Geometry check sheet. Reference: the model listing, model coordinates, mm. Coordinates: 2 decimals unless noted, no trailing zeros. Loops run counter-clockwise (first coordinate to the right, second up) from the corner with the lowest first, then second, coordinate; pieces in that order, holes last. Notation, with made-up numbers: (81.25, 34) - (112.25, 34) arc R12 cw to (112.25, 57) - close; hole circle Ø5 at (2.5, -29.75). An arc over 180 degrees is marked (long way). One line per item, written item: value.
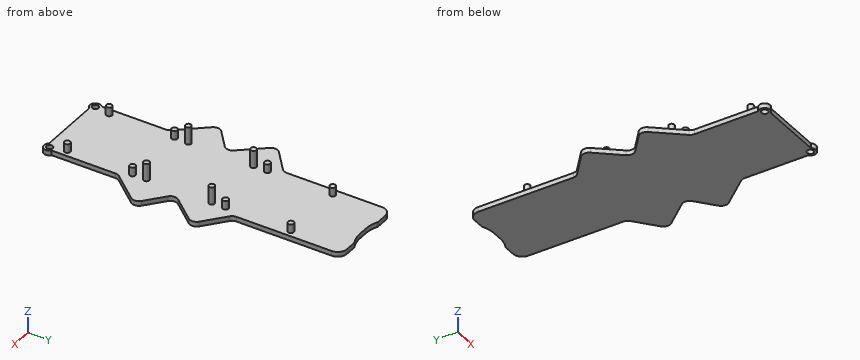
from build123d import *

# Parameters (mm, degrees)
F0_R     = 1.4859
F1_DEPTH = 2.2098
F2_R     = 1.33
F3_DEPTH = 4
F4_DEPTH = 8


with BuildPart() as f1:
    # F0 (on Top) → F1 (new body)
    with BuildSketch(Plane.XY):
        with BuildLine():
            Line((2.114807, 67.46875), (-2.114807, 67.46875))
            ThreePointArc((-2.114807, 67.46875), (-5.0139, 67.776541), (-7.783739, 68.686193))
            Line((-7.783739, 68.686193), (-8.215857, 68.880768))
            ThreePointArc((-8.215857, 68.880768), (-8.47063, 68.964439), (-8.737292, 68.99275))
            Line((-8.737292, 68.99275), (-13.69695, 68.99275))
            ThreePointArc((-13.69695, 68.99275), (-16.750237, 67.728037), (-18.01495, 64.67475))
            Line((-18.01495, 64.67475), (-18.01495, 20.943534))
            ThreePointArc((-18.01495, 20.943534), (-18.312512, 19.601529), (-19.149422, 18.511071))
            Line((-19.149422, 18.511071), (-28.620485, 10.56605))
            ThreePointArc((-28.620485, 10.56605), (-29.742839, 8.410727), (-29.01242, 6.09306))
            Line((-29.01242, 6.09306), (-20.055478, -4.584288))
            ThreePointArc((-20.055478, -4.584288), (-19.325058, -6.901955), (-20.447412, -9.057278))
            Line((-20.447412, -9.057278), (-28.620485, -15.91345))
            ThreePointArc((-28.620485, -15.91345), (-29.742839, -18.068773), (-29.01242, -20.38644))
            Line((-29.01242, -20.38644), (-18.757488, -32.611089))
            ThreePointArc((-18.757488, -32.611089), (-18.206354, -33.565901), (-18.01495, -34.651617))
            Line((-18.01495, -34.651617), (-18.01495, -63.949145))
            ThreePointArc((-18.01495, -63.949145), (-15.313338, -63.63877), (-13.864863, -65.940283))
            ThreePointArc((-13.864863, -65.940283), (-13.995237, -66.745649), (-14.373042, -67.46875))
            Line((-14.373042, -67.46875), (14.373042, -67.46875))
            ThreePointArc((14.373042, -67.46875), (14.643616, -64.104693), (18.01495, -63.949145))
            Line((18.01495, -63.949145), (18.01495, -34.651617))
            ThreePointArc((18.01495, -34.651617), (18.206354, -33.565901), (18.757488, -32.611089))
            Line((18.757488, -32.611089), (29.01242, -20.38644))
            ThreePointArc((29.01242, -20.38644), (29.742839, -18.068773), (28.620485, -15.91345))
            Line((28.620485, -15.91345), (20.447412, -9.057278))
            ThreePointArc((20.447412, -9.057278), (19.325058, -6.901955), (20.055478, -4.584288))
            Line((20.055478, -4.584288), (29.01242, 6.09306))
            ThreePointArc((29.01242, 6.09306), (29.742839, 8.410727), (28.620485, 10.56605))
            Line((28.620485, 10.56605), (19.149422, 18.511071))
            ThreePointArc((19.149422, 18.511071), (18.312512, 19.601529), (18.01495, 20.943534))
            Line((18.01495, 20.943534), (18.01495, 64.67475))
            ThreePointArc((18.01495, 64.67475), (16.750237, 67.728037), (13.69695, 68.99275))
            Line((13.69695, 68.99275), (8.737292, 68.99275))
            ThreePointArc((8.737292, 68.99275), (8.47063, 68.964439), (8.215857, 68.880768))
            Line((8.215857, 68.880768), (7.783739, 68.686193))
            ThreePointArc((7.783739, 68.686193), (5.0139, 67.776541), (2.114807, 67.46875))
        make_face()
        with BuildLine():
            ThreePointArc((-13.864863, -65.940283), (-15.313338, -63.63877), (-18.01495, -63.949145))
            ThreePointArc((-18.01495, -63.949145), (-18.19151, -67.775873), (-14.373042, -67.46875))
            ThreePointArc((-14.373042, -67.46875), (-13.995237, -66.745649), (-13.864863, -65.940283))
        make_face()
        with Locations((-16.417563, -65.940283)):
            Circle(F0_R, mode=Mode.SUBTRACT)
        with BuildLine():
            ThreePointArc((18.970263, -65.940283), (18.719076, -64.836058), (18.01495, -63.949145))
            ThreePointArc((18.01495, -63.949145), (14.643616, -64.104693), (14.373042, -67.46875))
            ThreePointArc((14.373042, -67.46875), (17.222929, -68.362609), (18.970263, -65.940283))
        make_face()
        with Locations((16.417563, -65.940283)):
            Circle(F0_R, mode=Mode.SUBTRACT)
    extrude(amount=F1_DEPTH)

    # F2 (on face) → F3 (join)
    with BuildSketch(Plane.XY.offset(2.2098)):
        with Locations((-15, 44.01575)):
            Circle(F2_R)
        with Locations((15, 44.01575)):
            Circle(F2_R)
        with Locations((15, 14.01575)):
            Circle(F2_R)
        with Locations((-15, 14.01575)):
            Circle(F2_R)
        with Locations((15, -28.68425)):
            Circle(F2_R)
        with Locations((-15, -28.68425)):
            Circle(F2_R)
        with Locations((-15, -58.68425)):
            Circle(F2_R)
        with Locations((15, -58.68425)):
            Circle(F2_R)
    extrude(amount=F3_DEPTH)

    # F2 (on face) → F4 (join)
    with BuildSketch(Plane.XY.offset(2.2098)):
        with Locations((15, 7.66575)):
            Circle(F2_R)
        with Locations((15, -22.33425)):
            Circle(F2_R)
        with Locations((-15, -22.33425)):
            Circle(F2_R)
        with Locations((-15, 7.66575)):
            Circle(F2_R)
    extrude(amount=F4_DEPTH)


solid = f1.part
(1) Cross-section at B-B on y = 37.5. Record the cut outline in (x, z), and give its area (3 significant figures).
Reply:
outline: (-18.01, 0) - (18.01, 0) - (18.01, 2.21) - (-18.01, 2.21) - close
area: 79.6 mm2
(2) Go/stop test with flat-tipped pins: pin 1 Ø2.5 at (x, z) = (5.5, 1.5) entering from -Y; pin 2 Ø0.8 at (x, y) = (-15, -29) entering from +Z; pin 3 Ø8 at (x, y) = (5, -32.5) entering from +Z. Record where each tip stops, or that it passes through.
Reply:
pin 1: y = -67.47
pin 2: z = 6.21
pin 3: z = 2.21
(3) Cross-section at C-C on x = 11.5. Record the cut outline in (y, z).
Reply:
outline: (-67.47, 0) - (68.99, 0) - (68.99, 2.21) - (-67.47, 2.21) - close
(4) Cross-section at A-A on x = 26. Record the cut outline in (y, z), and give its area (3 significant figures).
Reply:
outline: (-23.98, 0) - (-13.72, 0) - (-13.72, 2.21) - (-23.98, 2.21) - close; (2.5, 0) - (12.76, 0) - (12.76, 2.21) - (2.5, 2.21) - close
area: 45.4 mm2
(5) Material ranges on probe 1 along Z at (x, y) = (6.5, 12); probe 2 along X at (y, z) = (8, 3.5); probe 3 along Z at (x, y) = (15.5, -27.5), recorded low to high. Write a range as from..to.
Reply:
probe 1: 0..2.21
probe 2: -16.29..-13.71, 13.71..16.29
probe 3: 0..6.21
